Input: dimensioned drawing with shaded views. Units: mm. Origin: part minimum x, y, z. A direction names the side the tool comes from. Coordinates: 2 decimals unless noted, no trailing zeros. Loops run counter-clockwise (first coordinate to the right, second up) from the corner with the lowest first, then second, coordinate; pieces in that order, holes last. Notation, with made-up numbers: (53.5, -16) - (89.5, -16) arc R24 cw to (89.5, 0) - close; hole circle Ø8 at (-31.5, 68). An arc over 180 degrees is marked (long way). Put each result on its own line as item: value. Start each with the question number.
1) Contact query for flat-ended pins moving along their axis: pin 1 Ø6.5 at (y, z) = (14, 11) entering from -X; pin 2 Ø4 at (x, z) = (77.5, 12.5) entering from -Y; pin 3 Ø8 at (x, y) = (52, 11) entering from +Z. Output: stop coordinate, or through.
2) Section C-C on y = 11. Output: boundary loops of the cut face in (x, z), and give its area (3 significant figures).
3) Draft query along X for the marked faces 1, 2, 3 and 4. Return one class per face: +X half, -X half, draft (parallel to the pull), parting line (faces both ways), or undercut.
4) Section B-B on x = 33. Output: boundary loops of the cut face in (y, z), and give its area (3 significant figures).
5) Section A-A on z = 8.75. Output: boundary loops of the cut face in (x, y).
6) Reachability of the marked faces 5, 6 and 7 from +Z, -Z, +X, -X, +Y, -Y: full face, straight path, thin tool, end or side. Return the list, or none.
7) Section D-D on z = 1. Output: boundary loops of the cut face in (x, y), and give its area (3 significant figures).
8) Material intervals for line 1 along Y through (x, z) = (22, 14.5); line 2 along Y through (x, z) = (31, 2.5); line 3 along X through (y, z) = (19, 3.5), sorted ascending. Write a range as from..to.
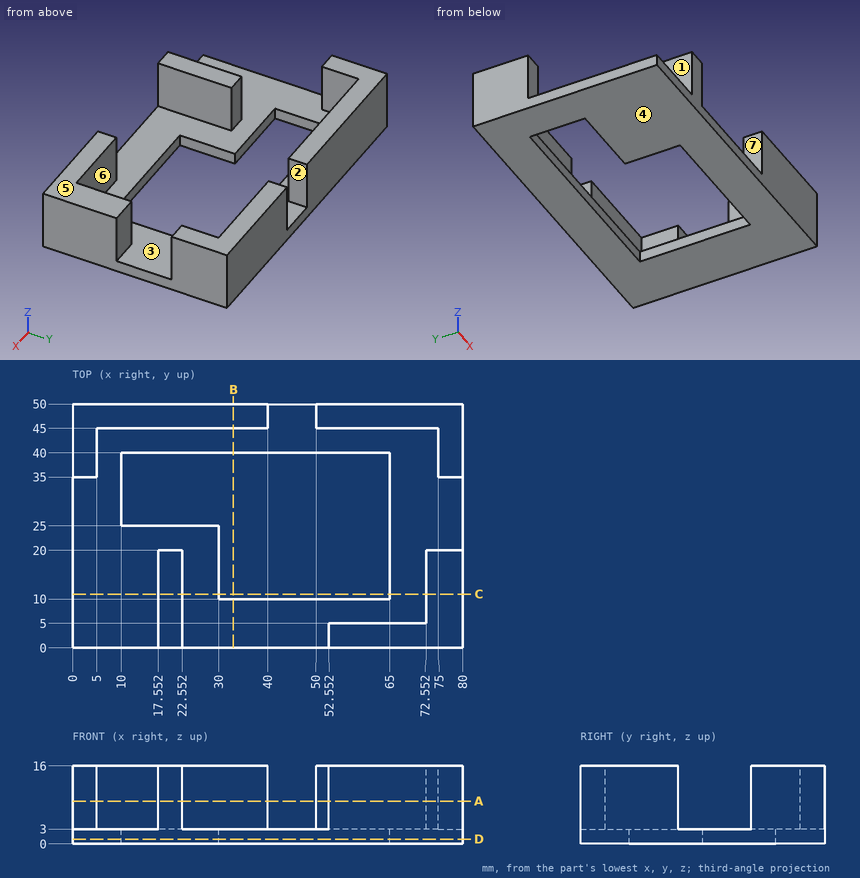
Answer block:
1. pin 1: stops at x = 17.55
1. pin 2: stops at y = 0
1. pin 3: stops at z = 3
2. outline: (0, 0) - (30, 0) - (30, 3) - (22.55, 3) - (22.55, 16) - (17.55, 16) - (17.55, 3) - (0, 3) - close; (65, 0) - (80, 0) - (80, 16) - (72.55, 16) - (72.55, 3) - (65, 3) - close
2. area: 297 mm²
3. face 1: -X half
3. face 2: undercut
3. face 3: undercut
3. face 4: draft
4. outline: (0, 0) - (10, 0) - (10, 3) - (0, 3) - close; (40, 0) - (50, 0) - (50, 16) - (45, 16) - (45, 3) - (40, 3) - close
4. area: 125 mm²
5. outline: (0, 35) - (5, 35) - (5, 45) - (40, 45) - (40, 50) - (0, 50) - close; (17.55, 0) - (22.55, 0) - (22.55, 20) - (17.55, 20) - close; (50, 45) - (75, 45) - (75, 35) - (80, 35) - (80, 50) - (50, 50) - close; (52.55, 0) - (80, 0) - (80, 20) - (72.55, 20) - (72.55, 5) - (52.55, 5) - close
6. face 5: +Z, +X, -X, +Y, -Y
6. face 6: +Z
6. face 7: +Z, -Y
7. outline: (0, 0) - (80, 0) - (80, 50) - (0, 50) - close; hole (10, 25) - (30, 25) - (30, 10) - (65, 10) - (65, 40) - (10, 40) - close
7. area: 2,650 mm²
8. line 1: y = 0..20, 45..50
8. line 2: y = 0..10, 40..50
8. line 3: x = 17.55..22.55, 72.55..80
